from build123d import *

# Parameters (mm, degrees)
F1_DEPTH = 12
F3_D     = 9
F3_DEPTH = 12
F3_TIP   = 2.7038727856
F5_D     = 9
F5_DEPTH = 12
F5_TIP   = 2.7038727856
F7_D     = 9
F7_DEPTH = 12
F7_TIP   = 2.7038727856
F8_R     = 15
F9_DEPTH = 0.5


with BuildPart() as f1:
    # F0 (on Front) → F1 (new body)
    with BuildSketch(Plane.XZ):
        Polygon((2.5, 23), (0, 23), (-2.5, 23), (-13.5460582414, 18.3112264581), (-6, 0), (0, 0), (6, 0), (13.5460582414, 18.3112264581), align=None)
    extrude(amount=F1_DEPTH)

    # F3
    with Locations(Plane(origin=(0, 0, 0), x_dir=(1, 0, 0), z_dir=(0, 0, -1))):
        with Locations((0, 6)):
            Hole(F3_D / 2, depth=F3_DEPTH)
            with Locations((0, 0, -(F3_DEPTH + F3_TIP / 2))):  # 118° drill point
                Cone(0, F3_D / 2, F3_TIP, mode=Mode.SUBTRACT)

    # F5
    with Locations(Plane(origin=(8.6540847408, 0, 20.3877460107), x_dir=(0.9205048535, 0, -0.3907311285), z_dir=(0.3907311285, 0, 0.9205048535))):
        with Locations((-0.6855538216, -6)):
            Hole(F5_D / 2, depth=F5_DEPTH)
            with Locations((0, 0, -(F5_DEPTH + F5_TIP / 2))):  # 118° drill point
                Cone(0, F5_D / 2, F5_TIP, mode=Mode.SUBTRACT)

    # F7
    with Locations(Plane(origin=(-8.6540847408, 0, 20.3877460107), x_dir=(0.9205048535, 0, 0.3907311285), z_dir=(-0.3907311285, 0, 0.9205048535))):
        with Locations((0.6855538216, -6)):
            Hole(F7_D / 2, depth=F7_DEPTH)
            with Locations((0, 0, -(F7_DEPTH + F7_TIP / 2))):  # 118° drill point
                Cone(0, F7_D / 2, F7_TIP, mode=Mode.SUBTRACT)

    # F8 (on face) → F9 (join)
    with BuildSketch(Plane(origin=(0, 0, 0), x_dir=(-1, 0, 0), z_dir=(0, 1, 0))):
        with Locations((0, 13)):
            Circle(F8_R)
    extrude(amount=F9_DEPTH)


solid = f1.part
Geometry check sheet. Reference: the model listing, model coordinates, mm. A direction names the side the tool comes from. Coordinates: 2 decimals unless noted, no trailing zeros. Order: outer loops, then holes, each group sorted by start corner. A loop starts at its lowest first (then second) coordinate and runs counter-clockwise, first axis right, second up. Notation, with made-up numbers: (67, 8) - (90, 8) arc R31 cw to (90, 40) - close; hole circle Ø4 at (69.25, 64.5). An arc over 180 degrees is marked (long way). Answer in a Markdown table with one row per item. Add a question column.
1) Cross-section at A-A, the plane x = 12.75. Record the cut outline in (y, z), then the cut area to 3 significant figures.
2) Material ranges on line 1 along Y through (x, z) = (0, 7); line 2 along Y through (x, z) = (11, 8); line 3 along Y through (x, z) = (6, 20.75), recorded low to high. Write a range as [from, to].
3) Gauge pin test, flat ends, axial feed: P1, Ø10, axis at x = 11, z = 6.5, coming from the -Y side; P2, Ø6, axis at x = -1, y = -3.5, coming from the -Z side; P3, Ø4, axis at y = -1, z = 5.5, coming from the +X side; P4, Ø2, axis at x = 11, z = 8.5, coming from the -Y side. Record the tip position at first contact, or that the pin passes through.
4) Set-up check for faces 4 (the flat face through (0, -6, 23)), 5 (the flat face through (-3, 0, 23)), 6 (the flat face through (-9.826, -5.916, 9.284)), 7 (the flat face through (9.72, -5.92, 9.03)): record each of +Z, -Z, +X, -X, +Y, -Y from which the full face is reachable in a straight line by a thin tool's end or side.
5) Cross-section at B-B, the plane y = -4.5. State how many separate pieces and enclosed holes the cut face has, then the cut area to 3 significant figures.
6) Cross-section at D-D, the plane z = 24. Record the cut outline in (x, y).
7) Release check for a two-part mould opening along X. For faces 1 (the flat face through (0, 0.5, 13)), 2 (the conical face through (5.015, -6.065, 7.506)), 3 (the flat face through (-11.628, -3.249, 19.126)) record: +X half, -X half, draft (parallel to the pull), parting line (faces both ways), or undercut.
Check result:
| question | item | result |
|---|---|---|
| 1 | outline | (-12, 16.38) - (0, 16.38) - (0, 5.1) - (0.5, 5.1) - (0.5, 20.9) - (0, 20.9) - (0, 18.65) - (-12, 18.65) - close |
| 1 | area | 35.1 mm² |
| 2 | line 1 | y = [-12, -10.5], [-1.5, 0.5] |
| 2 | line 2 | y = [0, 0.5] |
| 2 | line 3 | y = [-12, -10.08], [-1.92, 0.5] |
| 3 | P1 | stops at y = -12 |
| 3 | P2 | stops at z = 0 |
| 3 | P3 | stops at x = 13.85 |
| 3 | P4 | stops at y = 0 |
| 4 | face 4 | +Z, +X, -X, -Y |
| 4 | face 5 | -Y |
| 4 | face 6 | -Z, -X, -Y |
| 4 | face 7 | -Z, +X, -Y |
| 5 | separate pieces | 3 |
| 5 | enclosed holes | 0 |
| 5 | area | 139 mm² |
| 6 | outline | (-10.2, 0) - (10.2, 0) - (10.2, 0.5) - (-10.2, 0.5) - close |
| 7 | face 1 | draft |
| 7 | face 2 | undercut |
| 7 | face 3 | -X half |
